from build123d import *

# Parameters (mm, degrees)
MAIN_W                 = 46.736
MAIN_H                 = 1689.1
EXTRUDE_MAIN_DEPTH     = 44.45
MAIN_CUT_W             = 37.338
MAIN_CUT_H             = 39.37
CUT_MAIN_DEPTH         = 1690.846346839
BOTTOM_LEFT_W          = 26.67
BOTTOM_LEFT_H          = 2.667
CUT_BOTTOM_LEFT_DEPTH  = 1690.846346839
BOTTOM_RIGHT_W         = 6.096
BOTTOM_RIGHT_H         = 2.667
CUT_BOTTOM_RIGHT_DEPTH = 1690.846346839
LEFT_BOTTOM_W          = 3.048
LEFT_BOTTOM_H          = 6.858
CUT_LEFT_BOTTOM_DEPTH  = 1690.846346839
LEFT_MIDDLE_W          = 3.048
LEFT_MIDDLE_H          = 30.48
CUT_LEFT_MID_DEPTH     = 1690.846346839
RIGHT_MIDDLE_W         = 7.874
RIGHT_MIDDLE_H         = 28.702
CUT_RIGHT_MID_DEPTH    = 1690.846346839
HOOK_CUT_DEPTH         = 1690.846346839
FILLET3_R              = 1.905
FILLET4_R              = 0.508
SCREW_HOLES_D          = 5.3086


with BuildPart() as part:
    # Main → Extrude-Main (new body)
    with BuildSketch(Plane(origin=(0, 0, 0), x_dir=(1, 0, 0), z_dir=(0, 1, 0))):
        Rectangle(MAIN_W, MAIN_H)
    extrude(amount=EXTRUDE_MAIN_DEPTH)

    # Main Cut → Cut-Main (cut, through all)
    with BuildSketch(Plane.XY.offset(844.55)):
        with Locations((-4.699, 24.765)):
            Rectangle(MAIN_CUT_W, MAIN_CUT_H)
    extrude(amount=-CUT_MAIN_DEPTH, mode=Mode.SUBTRACT)

    # Bottom Left → Cut-Bottom Left (cut, through all)
    with BuildSketch(Plane.XY.offset(844.55)):
        with Locations((-7.493, 3.7465)):
            Rectangle(BOTTOM_LEFT_W, BOTTOM_LEFT_H)
    extrude(amount=-CUT_BOTTOM_LEFT_DEPTH, mode=Mode.SUBTRACT)

    # Bottom Right → Cut-Bottom Right (cut, through all)
    with BuildSketch(Plane.XY.offset(844.55)):
        with Locations((10.922, 3.7465)):
            Rectangle(BOTTOM_RIGHT_W, BOTTOM_RIGHT_H)
    extrude(amount=-CUT_BOTTOM_RIGHT_DEPTH, mode=Mode.SUBTRACT)

    # Left Bottom → Cut-Left Bottom (cut, through all)
    with BuildSketch(Plane.XY.offset(844.55)):
        with Locations((15.494, 5.842)):
            Rectangle(LEFT_BOTTOM_W, LEFT_BOTTOM_H)
    extrude(amount=-CUT_LEFT_BOTTOM_DEPTH, mode=Mode.SUBTRACT)

    # Left Middle → Cut-Left Mid (cut, through all)
    with BuildSketch(Plane.XY.offset(844.55)):
        with Locations((15.494, 26.730206209)):
            Rectangle(LEFT_MIDDLE_W, LEFT_MIDDLE_H)
    extrude(amount=-CUT_LEFT_MID_DEPTH, mode=Mode.SUBTRACT)

    # Right Middle → Cut-Right Mid (cut, through all)
    with BuildSketch(Plane.XY.offset(844.55)):
        with Locations((23.368, 22.225)):
            Rectangle(RIGHT_MIDDLE_W, RIGHT_MIDDLE_H)
    extrude(amount=-CUT_RIGHT_MID_DEPTH, mode=Mode.SUBTRACT)

    # Hooks → Hook Cut (cut, through all)
    with BuildSketch(Plane.XY.offset(844.55)):
        Polygon((19.431, 44.45), (19.431, 38.1635), (21.7805, 38.1635), (21.7805, 41.402), (23.368, 41.402), (23.368, 44.45), align=None)
        Polygon((23.368, 3.048), (23.368, 0), (19.431, 0), (19.431, 6.2865), (21.7805, 6.2865), (21.7805, 3.048), align=None)
    extrude(amount=-HOOK_CUT_DEPTH, mode=Mode.SUBTRACT)

    # Fillet3
    fillet3_edges = [part.edges().sort_by_distance(p)[0] for p in [
        (19.431, 44.45, 0),
        (19.431, 0, 0),
        (-23.368, 0, 0),
    ]]
    fillet(fillet3_edges, radius=FILLET3_R)

    # Fillet4
    fillet4_edges = [part.edges().sort_by_distance(p)[0] for p in [
        (23.368, 41.402, 0),
        (21.7805, 41.402, 0),
        (21.7805, 3.048, 0),
        (23.368, 3.048, 0),
        (-23.368, 5.08, 0),
        (13.97, 44.45, 0),
        (-20.828, 5.08, 0),
        (5.842, 5.08, 0),
        (7.874, 5.08, 0),
        (13.97, 9.271, 0),
        (13.97, 11.490206209, 0),
        (13.97, 41.970206209, 0),
        (23.368, 36.576, 0),
        (23.368, 7.874, 0),
    ]]
    fillet(fillet4_edges, radius=FILLET4_R)

    # Screw Holes (through all)
    with Locations(Plane.ZY.offset(-17.018)):
        with Locations((-791.21, 26.730206209), (831.85, 26.730206209), (791.21, 26.730206209), (-831.85, 26.730206209)):
            Hole(SCREW_HOLES_D / 2)


solid = part.part
Design review of the part built by this model. Coordinates are the model's own, in mm. A direction names the side the tool comes from. Coordinates: 2 decimals unless noted, no trailing zeros. Order: outer loops, then holes, each group sorted by start corner. A loop starts at its lowest first (then second) coordinate and runs counter-clockwise, first axis right, second up.
Item 1: Take a section at A-A, the plane x = -12. Write out the cut boundary in (y, z).
Item 2: For faces 4 (the flat face through (17.2, 13.9, 844.55)), 5 (the flat face through (17.018, 27, 12)), 6 (the flat face through (-8, 2.413, 12)), list the 3-axis set-ups (+Z, -Z, +X, -X, +Y, -Y) from which the entire face can be reached by the end or side of a thin tool; tool diameter is ignored.
Item 3: The part is to be moulded in two halves that separate along Y. For faces 1 (the flat face through (19.431, 22, 12)), 2 (the flat face through (-2, 0, -12)), 3 (the flat face through (17.2, 13.9, -844.55)), say which applies: pulls with the +Y half, pulls with the -Y half, needs draft (parallel to the pull), parting line crosses it, or undercut.
Item 4: For line 1 (X direction, y = 5, z = 219.5); line 2 (Y direction, x = 17.9, z = 831.85); line 3 (Y direction, x = 18, z = 791), list the stretches that pass through material, from the lowest coordinate up.
Item 5: For pin 1 Ø13.5 at (x, z) = (-11.5, -317.5) entering from +Y; pin 2 Ø2 at (y, z) = (7.5, 249) entering from -X; pin 3 Ø0.5 at (x, z) = (7, 225) entering from +Y, all flat-tipped, find the tip position at first contact; note any pin that passes through.
The answers:
1. outline: (0, -844.55) - (2.41, -844.55) - (2.41, 844.55) - (0, 844.55) - close
2. face 4: +Z, +X, -X, +Y, -Y
2. face 5: +Z, -Z, -X
2. face 6: +Z, -Z, +Y
3. face 1: undercut
3. face 2: pulls with the -Y half
3. face 3: needs draft
4. line 1: x = -23.13 to -21.06, 6.08 to 7.64, 17.02 to 19.43, 21.78 to 23.37
4. line 2: y = 0.04 to 24.08, 29.38 to 44.41
4. line 3: y = 0.06 to 24.08, 29.38 to 44.39
5. pin 1: stops at y = 2.41
5. pin 2: stops at x = 17.02
5. pin 3: stops at y = 5.08
